Build history of the part. All positions in model axes, mm. A direction names the side the tool comes from. Round coordinates to 2 decimals unless told otherwise and drop trailing zeros. Loops run counter-clockwise (first coordinate to the right, second up) from the corner with the lowest first, then second, coordinate; pieces in that order, holes last. Notation, with made-up numbers: M 38.25,-3.75 L 93.25,-3.75 A10 ccw 93.25,5.25 Z; hole C 28.25,88.5 d9. An arc over 180 degrees is marked long. Use one line per item in the form item = value. Start each with the question number.
```python
from build123d import *

# Parameters (mm, degrees)
F0_R      = 56.9
F1_DEPTH  = 82.4
F2_R      = 6.55
F3_DEPTH  = 82.4
F4_R      = 56
F5_DEPTH  = 47.7
F6_R      = 42.9
F7_DEPTH  = 65.4
F8_R      = 23.8
F9_DEPTH  = 69.4
F10_R     = 12.75
F11_DEPTH = 71.2


with BuildPart() as f1:
    # F0 (on Top) → F1 (new body)
    with BuildSketch(Plane.XY):
        Circle(F0_R)
    extrude(amount=F1_DEPTH)

    # F2 (on Top) → F3 (cut)
    with BuildSketch(Plane.XY):
        Circle(F2_R)
    extrude(amount=F3_DEPTH, mode=Mode.SUBTRACT)

    # F4 (on Top) → F5 (cut)
    with BuildSketch(Plane.XY):
        Circle(F4_R)
    extrude(amount=F5_DEPTH, mode=Mode.SUBTRACT)

    # F6 (on Top) → F7 (cut)
    with BuildSketch(Plane.XY):
        Circle(F6_R)
    extrude(amount=F7_DEPTH, mode=Mode.SUBTRACT)

    # F8 (on Top) → F9 (cut)
    with BuildSketch(Plane.XY):
        Circle(F8_R)
    extrude(amount=F9_DEPTH, mode=Mode.SUBTRACT)

    # F10 (on Top) → F11 (cut)
    with BuildSketch(Plane.XY):
        Circle(F10_R)
    extrude(amount=F11_DEPTH, mode=Mode.SUBTRACT)


solid = f1.part
```
Q1. Tool access for faces 5 (the face through (-31.62, 28.99, 56.43)), 6 (the face through (-1, -12, 82.4)): list every direction of +Z, -Z, +X, -X, +Y, -Y with a clear straight run to the whole face (end or side of a thin tool).
Q2. Drop flat-ended pins along their axis: P1, Ø1, axis at y = 16, z = 56.5, coming from the +X side; P2, Ø5, axis at y = 22, z = 15, coming from the +X side; P3, Ø2, axis at x = 23.5, y = 16, coming from the -Z side. Give the stop position or say it passes through.
Q3. Saw through at C-C (z = 36). Give the cut face in (x, y).
Q4. Wall check: probe 1 along Y at (x, z) = (0, 70.4); probe 2 along Y at (x, z) = (0, 38); probe 3 along X at (y, z) = (19.5, 44.5). Give the ranges that are in metal, low to high.
Q5. Pull direction Y, two halves, no side cores. Call faces 1 (the face through (10, -10, 69.4)), 2 (the face through (-12.7, -41.2, 47.7)), 3 (the face through (54.272, 17.091, 40.623)), 4 (the face through (42, -38, 0)): pulls with the +Y half, pulls with the -Y half, needs draft (parallel to the pull), parting line crosses it, or undercut.
Q6. Saw through at D-D (y = 50). Give the cut face in (x, z).
Q7. Saw through at A-A (y = 0). Give the cut face in (x, z).
Filled in:
q1.face_5 = -Z
q1.face_6 = +Z, +X, -X, +Y, -Y
q2.P1 = 54.75
q2.P2 = 53.45
q2.P3 = 65.4
q3.outline = C 0,0 d113.8; hole C 0,0 d112
q4.probe_1 = -56.9 to -12.75, 12.75 to 56.9
q4.probe_2 = -56.9 to -56, 56 to 56.9
q4.probe_3 = -53.45 to -52.5, 52.5 to 53.45
q5.face_1 = undercut
q5.face_2 = undercut
q5.face_3 = parting line crosses it
q5.face_4 = needs draft
q6.outline = M -27.16,0 L -25.22,0 L -25.22,47.7 L 25.22,47.7 L 25.22,0 L 27.16,0 L 27.16,82.4 L -27.16,82.4 Z
q7.outline = M -56.9,0 L -56,0 L -56,47.7 L -42.9,47.7 L -42.9,65.4 L -23.8,65.4 L -23.8,69.4 L -12.75,69.4 L -12.75,71.2 L -6.55,71.2 L -6.55,82.4 L -56.9,82.4 Z; M 6.55,71.2 L 12.75,71.2 L 12.75,69.4 L 23.8,69.4 L 23.8,65.4 L 42.9,65.4 L 42.9,47.7 L 56,47.7 L 56,0 L 56.9,0 L 56.9,82.4 L 6.55,82.4 Z
